Geometry check sheet. Reference: the model listing, model coordinates, mm. Face numbers are marked on the shaded views. A direction names the side the tool comes from. Round coordinates to 2 decimals unless told otherwise and drop trailing zeros. Loops run counter-clockwise (first coordinate to the right, second up) from the corner with the lowest first, then second, coordinate; pieces in that order, holes last. Notation, with made-up numbers: (69.5, 71.25) -> (76.5, 71.25) arc R11 ccw to (76.5, 81.25) -> close; hole circle Ø11 at (28, 21.5). An arc over 180 degrees is marked (long way). Use a Markdown table: item, result. Add a question column.
Q1. Gauge pin test, flat ends, axial feed: P1, Ø0.5, axis at x = -0.5, z = 33.5, coming from the +Y side; P2, Ø5, axis at x = 23, y = -2.5, coming from the +Z side; P3, Ø0.5, axis at x = -0.5, z = 33, coming from the -Y side. Record the tip position at first contact, or that the pin passes through.
Q2. Material ranges on L1, parallel to Z at x = 18, y = -4.5; L2, parallel to X at y = -2.75, z = 45.5; L3, parallel to X at y = -6.25, z = 32, recorded low to high.
Q3. Set-up check for the marked faces 1, 2 and 3: record each of +Z, -Z, +X, -X, +Y, -Y from which the full face is reachable in a straight line by a thin tool's end or side.
Q4. Sectioned sample at A-A, the plane z = 48. Enter the section's corners in (x, y), then the cut area to 3 significant figures.
```python
from build123d import *

# Parameters (mm, degrees)
F0_W     = 37
F0_H     = 53
F1_DEPTH = 12
F2_R     = 2
F4_R     = 1.5
F5_DEPTH = 5


with BuildPart() as f1:
    # F0 (on Front) → F1 (new body)
    with BuildSketch(Plane.XZ):
        with Locations((18.5, 26.5)):
            Rectangle(F0_W, F0_H)
        with BuildLine():
            ThreePointArc((37, 53), (18.5, 55), (0, 53))
            Line((0, 53), (37, 53))
        make_face()
    extrude(amount=F1_DEPTH)

    # F2
    f2_edges = [f1.edges().sort_by_distance(p)[0] for p in [
        (37, -6, 53),
        (18.5, -12, 55),
        (0, -6, 53),
        (18.5, 0, 55),
        (37, -12, 26.5),
        (37, 0, 26.5),
        (37, -6, 0),
        (18.5, -12, 0),
        (0, -12, 26.5),
        (0, 0, 26.5),
        (18.5, 0, 0),
        (0, -6, 0),
    ]]
    fillet(f2_edges, radius=F2_R)

    # F4 (on offset) → F5 (join, symmetric)
    with BuildSketch(Plane.XZ.offset(6)):
        with Locations((0, 33)):
            Circle(F4_R)
    extrude(amount=F5_DEPTH, both=True)


solid = f1.part
```
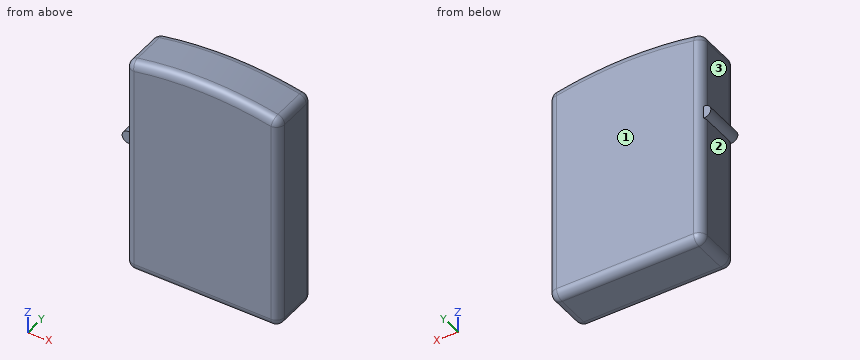
Values:
| question | item | result |
|---|---|---|
| 1 | P1 | y = -1 |
| 1 | P2 | z = 54.98 |
| 1 | P3 | y = -11 |
| 2 | L1 | 0 to 55 |
| 2 | L2 | 0 to 37 |
| 2 | L3 | -1.12 to 37 |
| 3 | face 1 | +Z, -Z, +X, -X, +Y |
| 3 | face 2 | -Z, -X, +Y, -Y |
| 3 | face 3 | +Z, -X, +Y, -Y |
| 4 | outline | (0, -10) arc R2 ccw to (2, -12) -> (35, -12) arc R2 ccw to (37, -10) -> (37, -2) arc R2 ccw to (35, 0) -> (2, 0) arc R2 ccw to (0, -2) -> close |
| 4 | area | 441 mm^2 |
